The figure shows three views and two pictorial views of one solid part (mm, origin at its lowest corner). Answer the questions. A direction names the side the tool comes from. Coordinates: 2 decimals unless noted, no trailing zeros. Order: outer loops, then holes, each group sorted by start corner. A loop starts at its lowest first (then second) coordinate and runs counter-clockwise, first axis right, second up. Notation, with made-up numbers: (58.25, -26.5) -> (83.25, -26.5) arc R37 ccw to (83.25, 11.5) -> close; hole circle Ø7 at (60.25, 46). An arc over 180 degrees is marked (long way). Return JSON: item names as keys, results as strings.
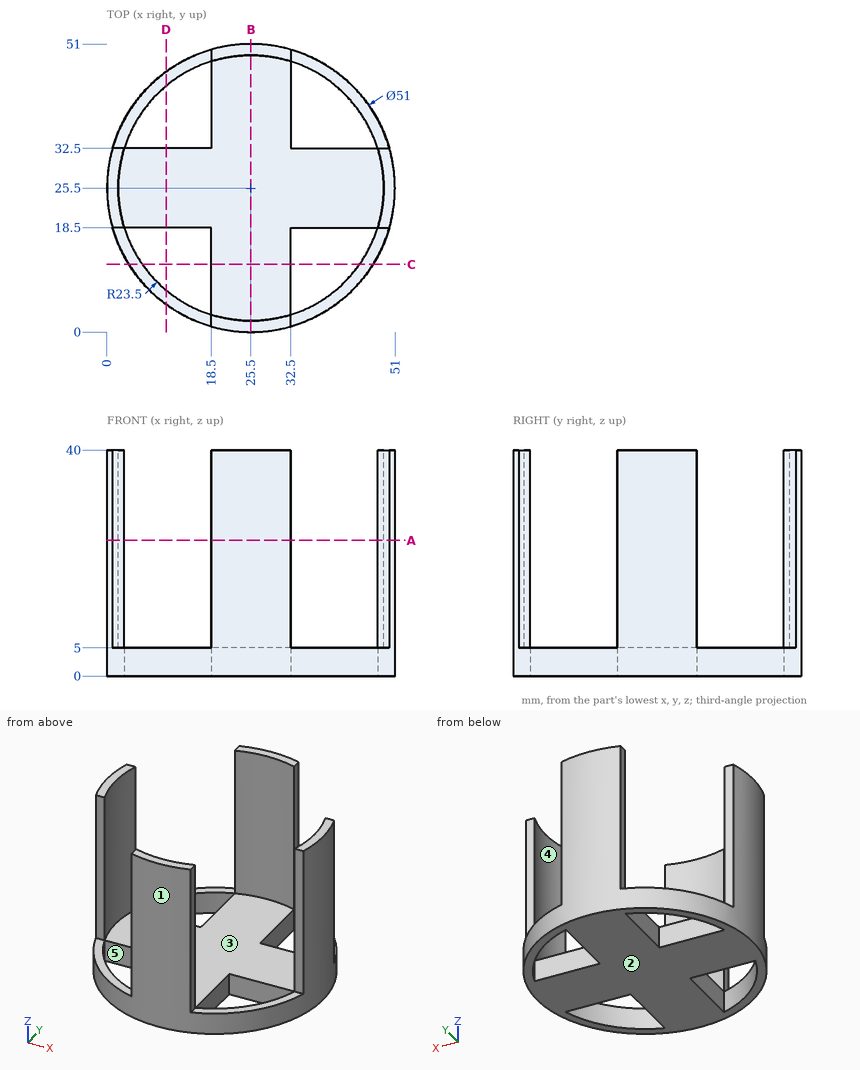
Item 1: Which of the six approach directions +Z, -Z, +X, -X, +Y, -Y give full straight-line access (tool end or side, diameter ignored) to the marked faces 4 and 5?
Answer list:
{"face 4": "+Z", "face 5": "+Z, -Z"}
Item 2: Flat-ended cylindrical pins translate along their axes: pin 1 (6 mm diameter, centred on x = 8.5, z = 32.5, fed in from +Y); pin 2 (10 mm diameter, centred on x = 38.5, z = 9.5, fed in from -Y); pin 3 (1.7 mm diameter, centred on y = 1.5, z = 16.5, fed in from +X); pin 4 (2.5 mm diameter, centred on x = 14, z = 2, fed in from +Y). Find the tip coordinate at first contact, or state that the pin passes through.
Answer list:
{"pin 1": "through", "pin 2": "y = 2.41", "pin 3": "x = 32.5", "pin 4": "y = 48.85"}
Item 3: The part is cut by section B-B on x = 25.5. Determine the outline of the cut face in (y, z).
Answer list:
{"outline": "(0, 0) -> (51, 0) -> (51, 40) -> (49, 40) -> (49, 5) -> (2, 5) -> (2, 40) -> (0, 40) -> close"}
Item 4: Determine the mould class of the marked faces 1, 2 and 3 for opening direction Y: pulls with the +Y half, pulls with the -Y half, needs draft (parallel to the pull), parting line crosses it, or undercut.
Answer list:
{"face 1": "parting line crosses it", "face 2": "needs draft", "face 3": "undercut"}
Item 5: The part is cut by section D-D on x = 10.5. Determine the outline of the cut face in (y, z).
Answer list:
{"outline": "(4.88, 0) -> (7.41, 0) -> (7.41, 5) -> (4.88, 5) -> close; (18.5, 0) -> (32.5, 0) -> (32.5, 5) -> (18.5, 5) -> close; (43.59, 0) -> (46.12, 0) -> (46.12, 5) -> (43.59, 5) -> close"}
Item 6: The part is cut by section C-C on y = 12. Determine the outline of the cut face in (x, z).
Answer list:
{"outline": "(3.87, 0) -> (6.26, 0) -> (6.26, 5) -> (3.87, 5) -> close; (18.5, 0) -> (32.5, 0) -> (32.5, 5) -> (18.5, 5) -> close; (44.74, 0) -> (47.13, 0) -> (47.13, 5) -> (44.74, 5) -> close"}
Item 7: Find the intervals of material crossed by probe 1 along X at (y, z) = (45.5, 3.5); probe 2 along Y at (x, z) = (25, 21.5); probe 3 along X at (y, z) = (36.5, 2), in increasing order.
Answer list:
{"probe 1": "9.68 to 13.16, 18.5 to 32.5, 37.84 to 41.32", "probe 2": "0 to 2.01, 48.99 to 51", "probe 3": "2.49 to 4.73, 18.5 to 32.5, 46.27 to 48.51"}
Item 8: The part is cut by section A-A on z = 24. Determine the outline of the cut face in (x, y).
Answer list:
{"outline": "(0.98, 18.5) -> (3.07, 18.5) arc R23.5 cw to (3.07, 32.5) -> (0.98, 32.5) arc R25.5 ccw to start; (18.5, 0.98) arc R25.5 ccw to (32.5, 0.98) -> (32.5, 3.07) arc R23.5 cw to (18.5, 3.07) -> close; (18.5, 47.93) arc R23.5 cw to (32.5, 47.93) -> (32.5, 50.02) arc R25.5 ccw to (18.5, 50.02) -> close; (47.93, 18.5) -> (50.02, 18.5) arc R25.5 ccw to (50.02, 32.5) -> (47.93, 32.5) arc R23.5 cw to start"}
